Check sheet for the modelled part. Datum: model origin and axes. Units: mm. Give positions to 0.01 mm unless a question says otherwise; leave off trailing zeros. Write each loop counter-clockwise with the first axis right and the second up, starting at its lowest first coordinate (ties: lowest second). Pieces come first, ordered by that corner, then holes.
from build123d import *

# Parameters (mm, degrees)
F0_W     = 127
F0_H     = 101.6
F1_DEPTH = 19.05
F2_R     = 3.175
F3_DEPTH = 25.4
F4_R     = 6.35
F5_DEPTH = 25.4


with BuildPart() as f1:
    # F0 (on Top) → F1 (new body)
    with BuildSketch(Plane.XY):
        Rectangle(F0_W, F0_H)
    extrude(amount=F1_DEPTH)

    # F2 (on face) → F3 (cut)
    with BuildSketch(Plane.XY.offset(19.05)):
        with Locations((-38.1, 25.4)):
            Circle(F2_R)
    extrude(amount=-F3_DEPTH, mode=Mode.SUBTRACT)

    # F4 (on face) → F5 (cut)
    with BuildSketch(Plane.XY.offset(19.05)):
        with Locations((12.7, -25.4)):
            Circle(F4_R)
    extrude(amount=-F5_DEPTH, mode=Mode.SUBTRACT)


solid = f1.part
1) Sectioned sample at A-A on y = 25.4. Record the boundary of the cut face in (x, z) (3 decimals), then the cut area to 3 significant figures.
2) Sectioned sample at B-B on x = -38.1. Record the boundary of the cut face in (y, z) (3 decimals).
3) Scan lines: L1, parallel to Y at x = 12.7, z = 12.5; L2, parallel to Y at x = -38.1, z = 10.75 (3 decimals); L3, parallel to X at y = 27, z = 11. Record each from-to range of solid material in increasing order.
4) Draft check along X on faces 1 (the cylindrical face through (7.66, -29.26, 9.66)), 2 (the flat face through (-1, 1, 19.05)), 3 (the flat face through (-63.5, -1, 9)). Enter one of: +X half, -X half, draft (parallel to the pull), parting line (faces both ways), or undercut.
Answers below:
1. outline: (-63.5, 0) - (-41.275, 0) - (-41.275, 19.05) - (-63.5, 19.05) - close; (-34.925, 0) - (63.5, 0) - (63.5, 19.05) - (-34.925, 19.05) - close
1. area: 2,300 mm2
2. outline: (-50.8, 0) - (22.225, 0) - (22.225, 19.05) - (-50.8, 19.05) - close; (28.575, 0) - (50.8, 0) - (50.8, 19.05) - (28.575, 19.05) - close
3. L1: y = -50.8 to -31.75, -19.05 to 50.8
3. L2: y = -50.8 to 22.225, 28.575 to 50.8
3. L3: x = -63.5 to -40.84, -35.36 to 63.5
4. face 1: undercut
4. face 2: draft
4. face 3: -X half
